from build123d import *

# Parameters (mm, degrees)
ESBO_O1_R                = 1.75
RESSALTO_EXTRUS_O1_DEPTH = 10
ESBO_O2_W                = 6
ESBO_O2_H                = 5
ESBO_O2_R                = 1.75
CORTE_EXTRUS_O1_DEPTH    = 10


with BuildPart() as part:
    # Esboço1 → Ressalto-extrusão1 (new body)
    with BuildSketch(Plane.XY):
        with BuildLine():
            Line((-5, 0), (-5, -20))
            Line((-5, -20), (5, -20))
            Line((5, -20), (5, 0))
            ThreePointArc((5, 0), (0, 5), (-5, 0))
        make_face()
        Circle(ESBO_O1_R, mode=Mode.SUBTRACT)
    extrude(amount=RESSALTO_EXTRUS_O1_DEPTH)

    # Esboço2 → Corte-extrusão1 (cut)
    with BuildSketch(Plane.ZY.offset(5)):
        with BuildLine():
            Line((10, 0), (4, 0))
            Line((4, 0), (4, -6.514718626))
            ThreePointArc((4, -6.514718626), (4.734013676, -8.824119703), (6.666666667, -10.285954792))
            ThreePointArc((6.666666667, -10.285954792), (9.082482905, -12.113248654), (10, -15))
            Line((10, -15), (10, 0))
        make_face()
        with Locations((7, 2.5)):
            Rectangle(ESBO_O2_W, ESBO_O2_H)
        with BuildLine():
            Line((10, -20), (10, -15))
            ThreePointArc((10, -15), (8.535533906, -18.535533906), (5, -20))
            Line((5, -20), (10, -20))
        make_face()
        with BuildLine():
            ThreePointArc((5, -20), (1.464466094, -18.535533906), (0, -15))
            Line((0, -15), (0, -20))
            Line((0, -20), (5, -20))
        make_face()
        with Locations((5, -15)):
            Circle(ESBO_O2_R)
    extrude(amount=-CORTE_EXTRUS_O1_DEPTH, mode=Mode.SUBTRACT)


solid = part.part
Design review of the part built by this model. Coordinates are the model's own, in mm. A direction names the side the tool comes from. Coordinates: 2 decimals unless noted, no trailing zeros. Order: outer loops, then holes, each group sorted by start corner. A loop starts at its lowest first (then second) coordinate and runs counter-clockwise, first axis right, second up. Notation, with made-up numbers: M 76,-34.5 L 89,-34.5 A23 ccw 89,-3.5 Z; hole C 8,-12 d5. An arc over 180 degrees is marked long. Use a Markdown table: item, result.
(1) Add section B-B (x = -3). Give the boundary of the cut face in (y, z).
Worked answers:
| item | result |
|---|---|
| outline | M -15,0 L 4,0 L 4,4 L -6.51,4 A4 cw -10.29,6.67 A5 ccw long Z; hole C -15,5 d3.5 |
(2) Wall thickness on probe 1 along Z at (x, y) = (-3.5, -0.75); probe 2 along Y at (x, z) = (-2.5, 5); probe 3 along Y at (x, z) = (0, 1.8): over which ranges is each line inside the solid? List them lowest first.
Worked answers:
| item | result |
|---|---|
| probe 1 | z = 0 to 4 |
| probe 2 | y = -20 to -16.75, -13.25 to -9.16 |
| probe 3 | y = -18.84 to -1.75, 1.75 to 5 |
(3) Add section D-D (z = 5.5). Give the boundary of the cut face in (x, y), then the cut area to 3 significant figures.
Worked answers:
| item | result |
|---|---|
| outline | M -5,-19.97 L 5,-19.97 L 5,-16.68 L -5,-16.68 Z; M -5,-13.32 L 5,-13.32 L 5,-9.64 L -5,-9.64 Z |
| area | 69.8 mm2 |
(4) Add section C-C (z = 1). Give the boundary of the cut face in (x, y), then the cut area to 3 significant figures.
Worked answers:
| item | result |
|---|---|
| outline | M -5,-18 L 5,-18 L 5,0 A5 ccw -5,0 Z; hole C 0,0 d3.5 |
| area | 210 mm2 |
(5) For faces 4 (the flat face through (0, -2, 4)), 5 (the flat face through (5, -12, 4)), list the 3-axis set-ups (+Z, -Z, +X, -X, +Y, -Y) from which the entire face can be reached by the end or side of a thin tool; tool diameter is ignored.
Worked answers:
| item | result |
|---|---|
| face 4 | +Z, +X, -X, +Y |
| face 5 | +Z, -Z, +X, +Y, -Y |
(6) Add section A-A (x = 0). Give the boundary of the cut face in (y, z), then the cut area to 3 significant figures.
Worked answers:
| item | result |
|---|---|
| outline | M -15,0 L -1.75,0 L -1.75,4 L -6.51,4 A4 cw -10.29,6.67 A5 ccw long Z; M 1.75,0 L 5,0 L 5,4 L 1.75,4 Z; hole C -15,5 d3.5 |
| area | 122 mm2 |
(7) For P1, Ø5, axis at x = 3.5, z = 4.5, coming from the +Y side; P2, Ø6, axis at x = -2, z = 6.5, coming from the +Y side; P3, Ø5, axis at x = -0.5, y = -1.5, coming from the +Z side, all flat-tipped, find the tip position at first contact; note any pin that passes through.
Worked answers:
| item | result |
|---|---|
| P1 | stops at y = 4.89 |
| P2 | stops at y = 4.99 |
| P3 | stops at z = 4 |
(8) Draft analysis for pull direction Y (two halves, no side actions). For faces 1 (the flat face through (0, -5, 0)), 2 (the cylindrical face through (1.617, -0.67, 1.972)), 3 (the cylindrical face through (-0.07, -8.796, 4.714)), state which applies: released by +Y, released by -Y, zero draft, split by the parting line, or undercut.
Worked answers:
| item | result |
|---|---|
| face 1 | zero draft |
| face 2 | undercut |
| face 3 | released by +Y |
